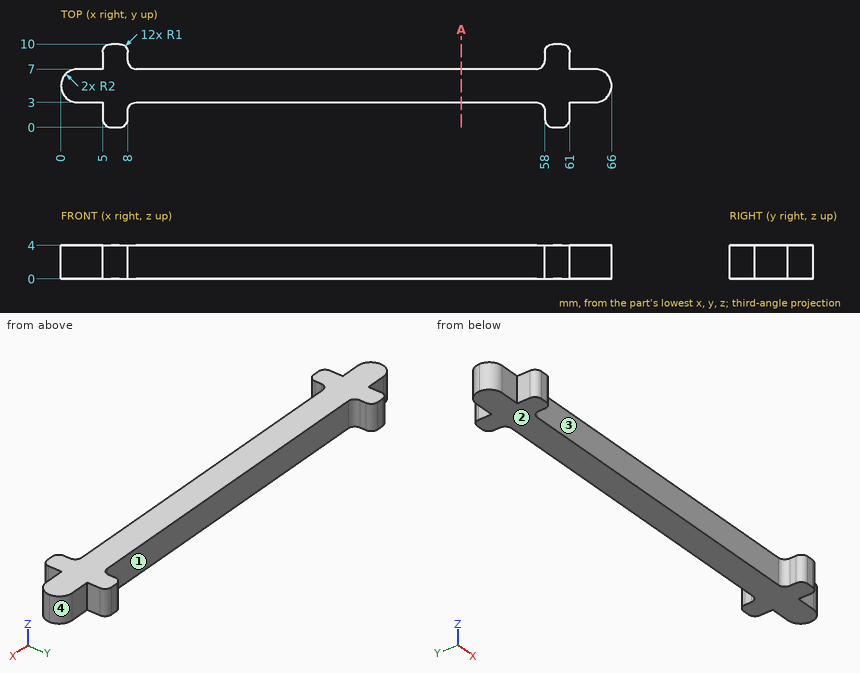
Input: dimensioned drawing with shaded views. Units: mm. Origin: part minimum x, y, z. Round coordinates to 2 decimals unless told otherwise and drop trailing zeros. Loops run counter-clockwise (first coordinate to the right, second up) from the corner with the lowest first, then second, coordinate; pieces in that order, holes last. Notation, with made-up numbers: M 54.25,7.25 L 76.25,7.25 A20 ccw 76.25,42.25 Z; hole C 66.5,-13 d6. An arc over 180 degrees is marked long. Answer in a Markdown table with one row per item. Add a question column.
1. Section A-A (x = 48). Output: boundary loops of the cut face in (y, z), and give its area (3 significant figures).
2. Ray query, probe 1 along X at (y, z) = (1.5, 2.2); probe 2 along Y at (x, z) = (30, 1.15); probe 3 along X at (y, z) = (7.5, 3.1). Return the intervals inside material, ascending.
3. Mould query, pull axis X, two halves, no side actions, for the marked faces 1, 2, 3 and 4. Classes: released by +X, released by -X, zero draft, split by the parting line, or undercut.
4. Contact query for flat-ended pins moving along their axis: pin 1 (0.8 mm diameter, centred on y = 1.5, z = 3, fed in from +X); pin 2 (1 mm diameter, centred on y = 1.5, z = 2.5, fed in from -X); pin 3 (1.5 mm diameter, centred on x = 62.5, z = 1.5, fed in from -Y). Output: stop coordinate, or through.
Values follow:
| question | item | result |
|---|---|---|
| 1 | outline | M 3,0 L 7,0 L 7,4 L 3,4 Z |
| 1 | area | 16.0 mm^2 |
| 2 | probe 1 | 5 to 8, 58 to 61 |
| 2 | probe 2 | 3 to 7 |
| 2 | probe 3 | 5 to 8.13, 57.87 to 61 |
| 3 | face 1 | undercut |
| 3 | face 2 | zero draft |
| 3 | face 3 | undercut |
| 3 | face 4 | released by +X |
| 4 | pin 1 | x = 61 |
| 4 | pin 2 | x = 5 |
| 4 | pin 3 | y = 3 |
